from build123d import *

# Parameters (mm, degrees)
F0_W     = 410
F0_H     = 150
F1_DEPTH = 16
F2_R     = 20
F3_DEPTH = 16.001
F4_R     = 63.5
F5_R     = 7.62


# Not quite as in the source:
# - a feature names something its author has since deleted; it is built from what else it names


with BuildPart() as f1:
    # F0 (on Top) → F1 (new body)
    with BuildSketch(Plane.XY):
        with Locations((-205, 75)):
            Rectangle(F0_W, F0_H)
    extrude(amount=F1_DEPTH)

    # F2 (on face) → F3 (cut, through all)
    with BuildSketch(Plane(origin=(0, 0, 0), x_dir=(1, 0, 0), z_dir=(0, 0, -1))):
        with Locations((-205, -75)):
            Circle(F2_R)
    extrude(amount=-F3_DEPTH, mode=Mode.SUBTRACT)

    # F4
    f4_edges = [f1.edges().sort_by_distance(p)[0] for p in [
        (-410, 150, 8),
        (-410, 0, 8),
        (0, 0, 8),
        (0, 150, 8),
    ]]
    fillet(f4_edges, radius=F4_R)

    # F5
    f5_edges = [f1.edges().sort_by_distance(p)[0] for p in [
        (-205, 0, 0),
        (-205, 0, 16),
        (-225, 75, 16),
        (-391.401281, 18.598719, 0),
        (-18.598719, 18.598719, 0),
        (-410, 75, 0),
        (0, 75, 0),
        (-391.401281, 131.401281, 0),
        (-18.598719, 131.401281, 0),
        (-205, 150, 0),
        (-225, 75, 0),
    ]]
    fillet(f5_edges, radius=F5_R)


solid = f1.part
Build history of the part. All positions in model axes, mm. Round coordinates to 2 decimals unless told otherwise and drop trailing zeros. Write each loop counter-clockwise with the first axis right and the second up, starting at its lowest first coordinate (ties: lowest second). Pieces come first, ordered by that corner, then holes. Notation, with made-up numbers: (15, 0) - (28, 0) arc R18 ccw to (28, 34) - close; hole circle Ø5 at (43.25, 3.5). An arc over 180 degrees is marked (long way). One line per question, with ' | ' between items.
1. Band-saw the part on A-A, the plane x = -205. Write the cut outline in (y, z), and give its area (3 significant figures).
Results are:
outline: (0, 7.62) arc R7.62 ccw to (7.62, 0) - (47.38, 0) arc R7.62 ccw to (55, 7.62) - (55, 8.38) arc R7.62 ccw to (47.38, 16) - (7.62, 16) arc R7.62 ccw to (0, 8.38) - close; (95, 7.62) arc R7.62 ccw to (102.62, 0) - (142.38, 0) arc R7.62 ccw to (150, 7.62) - (150, 8.38) arc R7.62 ccw to (142.38, 16) - (102.62, 16) arc R7.62 ccw to (95, 8.38) - close | area: 1,660 mm^2
2. Band-saw the part on C-C, the plane x = -87. Write the cut outline in (y, z), and give its area (3 significant figures).
Results are:
outline: (0, 7.62) arc R7.62 ccw to (7.62, 0) - (142.38, 0) arc R7.62 ccw to (150, 7.62) - (150, 8.38) arc R7.62 ccw to (142.38, 16) - (7.62, 16) arc R7.62 ccw to (0, 8.38) - close | area: 2,350 mm^2
3. Drill centre lines: line 1 along X through (y, z) = (75, 8.05); line 2 along Y through (x, z) = (-205, 7.8); line 3 along Y through (x, z) = (-124.5, 9.5). Where is each one in solid material? Low to high. Write a range as from..to.
Results are:
line 1: -410..-225, -185..0 | line 2: 0..55, 95..150 | line 3: 0.08..149.92
4. Drop flat-ended pins along their axis: pin 1 Ø2 at (y, z) = (25, 6) entering from +X; pin 2 Ø2 at (x, z) = (-235, 11.5) entering from +Y; pin 3 Ø6 at (y, z) = (21, 4.5) entering from -X. Give the stop position or say it passes through.
Results are:
pin 1: x = -12.43 | pin 2: y = 149.7 | pin 3: x = -395.7
5. Mould opens along Y. For faces 1 (the face through (-407.709, 74.839, 13.827)), 2 (the face through (-391.892, 130.905, 8.005)), 3 (the face through (-391.892, 19.095, 8.005)), 4 (the face through (-221, 87, 8)) say: released by +Y, released by -Y, zero draft, split by the parting line, or undercut.
Results are:
face 1: zero draft | face 2: released by +Y | face 3: released by -Y | face 4: undercut
6. Band-saw the part on B-B, the plane y = 75. Write the cut outline in (x, z), and give its area (3 significant figures).
Results are:
outline: (-410, 7.62) arc R7.62 ccw to (-402.38, 0) - (-232.62, 0) arc R7.62 ccw to (-225, 7.62) - (-225, 8.38) arc R7.62 ccw to (-232.62, 16) - (-402.38, 16) arc R7.62 ccw to (-410, 8.38) - close; (-185, 7.62) arc R7.62 ccw to (-177.38, 0) - (-7.62, 0) arc R7.62 ccw to (0, 7.62) - (0, 8.38) arc R7.62 ccw to (-7.62, 16) - (-177.38, 16) arc R7.62 ccw to (-185, 8.38) - close | area: 5,820 mm^2
